```python
from build123d import *

# Parameters (mm, degrees)
SKETCH_W               = 10.8
SKETCH_H               = 8.2
PAD_DEPTH              = 8.6
SKETCH001_W            = 3
SKETCH001_H            = 2
POCKET_DEPTH           = 10.801
LINEARPATTERN_COUNT    = 2
LINEARPATTERN_PITCH    = 3.8
POCKET001_DEPTH        = 8.601
SKETCH003_W            = 4.1
SKETCH003_H            = 2.8
POCKET002_DEPTH        = 9.501
LINEARPATTERN001_COUNT = 2
LINEARPATTERN001_PITCH = 3.8
SKETCH004_W            = 1
SKETCH004_H            = 7.6
POCKET003_DEPTH        = 9.501
SKETCH005_R            = 1.8
POCKET004_DEPTH        = 8.601
SKETCH006_R            = 4
PAD001_DEPTH           = 5
SKETCH007_R            = 1.8
POCKET005_DEPTH        = 5
CHAMFER_SIZE           = 0.5


with BuildPart() as part:
    # Sketch → Pad (new body)
    with BuildSketch(Plane.XZ):
        Rectangle(SKETCH_W, SKETCH_H)
    extrude(amount=-PAD_DEPTH)

    # Sketch001 (on Face2 of Pad) → Pocket (cut, through all)
    with BuildSketch(Plane(origin=(5.4, 0, 0), x_dir=(0, 0, 1), z_dir=(1, 0, 0))):
        with Locations((-2.6, -2.4)):
            Rectangle(SKETCH001_W, SKETCH001_H)
    pocket = extrude(amount=-POCKET_DEPTH, mode=Mode.SUBTRACT)

    # LinearPattern: Pocket ×2
    with Locations(*[(0, i * LINEARPATTERN_PITCH, 0) for i in range(1, LINEARPATTERN_COUNT)]):
        add(pocket, mode=Mode.SUBTRACT)

    # Sketch002 (on Face4 of LinearPattern) → Pocket001 (cut, through all)
    with BuildSketch(Plane.XZ):
        Polygon((-5.4, 0), (-4.1, 0), (-4.1, 4.1), (4.1, 4.1), (4.1, 0), (5.4, 0), (5.4, 5), (-5.4, 5), align=None)
    extrude(amount=-POCKET001_DEPTH, mode=Mode.SUBTRACT)

    # Sketch003 (on Face3 of Pocket001) → Pocket002 (cut, through all)
    with BuildSketch(Plane(origin=(4.1, 0, 0), x_dir=(0, 0, 1), z_dir=(1, 0, 0))):
        with Locations((2.05, -2.4)):
            Rectangle(SKETCH003_W, SKETCH003_H)
    pocket002 = extrude(amount=-POCKET002_DEPTH, mode=Mode.SUBTRACT)

    # LinearPattern001: Pocket002 ×2
    with Locations(*[(0, i * LINEARPATTERN001_PITCH, 0) for i in range(1, LINEARPATTERN001_COUNT)]):
        add(pocket002, mode=Mode.SUBTRACT)

    # Sketch004 (on Face25 of LinearPattern001) → Pocket003 (cut, through all)
    with BuildSketch(Plane(origin=(4.1, 0, 0), x_dir=(0, 0, 1), z_dir=(1, 0, 0))):
        with Locations((3.6, -4.8)):
            Rectangle(SKETCH004_W, SKETCH004_H)
    extrude(amount=-POCKET003_DEPTH, mode=Mode.SUBTRACT)

    # Sketch005 (on Face2 of Pocket003) → Pocket004 (cut, through all)
    with BuildSketch(Plane.XZ):
        Circle(SKETCH005_R)
    extrude(amount=-POCKET004_DEPTH, mode=Mode.SUBTRACT)

    # Sketch006 (on Face2 of Pocket004) → Pad001 (join)
    with BuildSketch(Plane.XZ):
        Circle(SKETCH006_R)
    extrude(amount=PAD001_DEPTH)

    # Sketch007 (on Face32 of Pad001) → Pocket005 (cut)
    with BuildSketch(Plane.XZ.offset(5)):
        Circle(SKETCH007_R)
    extrude(amount=-POCKET005_DEPTH, mode=Mode.SUBTRACT)

    # Chamfer
    chamfer_edges = [part.edges().sort_by_distance(p)[0] for p in [
        (-4, -5, 0),
    ]]
    chamfer(chamfer_edges, length=CHAMFER_SIZE)


solid = part.part
```
Can you work these out from the model? Positions are in its coordinate system, mm. A direction names the side the tool comes from. Coordinates: 2 decimals unless noted, no trailing zeros. Loops run counter-clockwise (first coordinate to the right, second up) from the corner with the lowest first, then second, coordinate; pieces in that order, holes last. Notation, with made-up numbers: (-36.75, 44) -> (-7.75, 44) arc R21 ccw to (-7.75, 62) -> close; hole circle Ø6 at (-8, 26.25). An arc over 180 degrees is marked (long way). Answer as a JSON object with one key per item and string values.
1) Imagine slicing it at C-C (x = 4.5). Please give me the cut outline in (y, z), then the cut area to 3 significant figures.
Results:
{"outline": "(0, -4.1) -> (1.4, -4.1) -> (1.4, -1.1) -> (3.4, -1.1) -> (3.4, -4.1) -> (5.2, -4.1) -> (5.2, -1.1) -> (7.2, -1.1) -> (7.2, -4.1) -> (8.6, -4.1) -> (8.6, 0) -> (0, 0) -> close", "area": "23.3 mm^2"}
2) If I drill on line 1 (Y direction, x = 1, z = -2.25); line 2 (Y direction, x = 4, z = 2.25); line 3 (Z direction, x = -2.5, y = 3), over which ranges is the centre line in solid material (lowest first)?
Results:
{"line 1": "y = -5 to 1.4, 3.4 to 5.2, 7.2 to 8.6", "line 2": "y = 0 to 1, 3.8 to 4.8, 7.6 to 8.6", "line 3": "z = -1.1 to 0"}
3) Imagine slicing it at B-B (y = 6.5). Please give me the cut outline in (x, z).
Results:
{"outline": "(-5.4, -1.1) -> (-1.42, -1.1) arc R1.8 cw to (-1.8, 0) -> (-5.4, 0) -> close; (1.42, -1.1) -> (5.4, -1.1) -> (5.4, 0) -> (1.8, 0) arc R1.8 cw to start"}
4) Imagine slicing it at D-D (y = -3.75). Please give me the cut outline in (x, z), then the cut area to 3 significant figures.
Results:
{"outline": "circle Ø8 at (0, 0); hole circle Ø3.6 at (0, 0)", "area": "40.1 mm^2"}
5) For P1, Ø1, axis at x = -4, z = -1, coming from the -Y side; P2, Ø0.8, axis at y = 0.5, z = 1.5, coming from the -X side; P3, Ø1.1, axis at y = 8, z = 1.5, coming from the +X side, each with a flat end and sliding along its axis, tell me the tip position at first contact or that it passes through.
Results:
{"P1": "stops at y = -4.88", "P2": "stops at x = -4.1", "P3": "stops at x = 4.1"}
6) Thinking about a two-plate mould opening in X: for faces 1 (the face through (0, 1, 2)), 2 (the face through (1.663, 1.705, -0.689)), 3 (the face through (4.1, 8, 2)), which applies, pulls with the +X half, pulls with the -X half, needs draft (parallel to the pull), parting line crosses it, or undercut?
Results:
{"face 1": "needs draft", "face 2": "undercut", "face 3": "pulls with the +X half"}
7) For faces 4 (the face through (-0.867, -2.218, -3.905)), 5 (the face through (0, 7.6, 2)), 6 (the face through (0, 3.4, -3)), 7 (the face through (0, 8, 3.1)), which set-ups out of +Z, -Z, +X, -X, +Y, -Y let a thin tool reach every point of the face, with its end or its side?
Results:
{"face 4": "-Y", "face 5": "+Z, +X, -X", "face 6": "-Z, +X, -X", "face 7": "+Z, +X, -X, +Y"}
8) Imagine slicing it at A-A (x = 0). Count the separate pieces of the cut face and the enclosed holes in it, then the cut area to 3 significant figures.
Results:
{"separate pieces": "6", "enclosed holes": "0", "area": "37.2 mm^2"}
